For this review, take the finished solid that the model builds, in its own axes (mm). A direction names the side the tool comes from. Round coordinates to 2 decimals unless told otherwise and drop trailing zeros. Order: outer loops, then holes, each group sorted by start corner. A loop starts at its lowest first (then second) coordinate and runs counter-clockwise, first axis right, second up.
```python
from build123d import *

# Parameters (mm, degrees)
F0_R     = 3.302
F1_DEPTH = 6.35


with BuildPart() as f1:
    # F0 (on Top) → F1 (new body)
    with BuildSketch(Plane.XY):
        with BuildLine():
            ThreePointArc((12.499722, -2.252856), (12.650669, -1.13092), (12.701119, 0))
            ThreePointArc((12.701119, 0), (12.700826, 0.086204), (12.699949, 0.172405))
            ThreePointArc((12.699949, 0.172405), (12.657421, 1.052668), (12.553954, 1.927863))
            ThreePointArc((12.553954, 1.927863), (12.311527, 3.121654), (11.955851, 4.28673))
            ThreePointArc((11.955851, 4.28673), (11.629806, 5.105489), (11.24777, 5.899668))
            ThreePointArc((11.24777, 5.899668), (10.630855, 6.95006), (9.916151, 7.936522))
            ThreePointArc((9.916151, 7.936522), (9.341922, 8.605052), (8.722716, 9.232153))
            ThreePointArc((8.722716, 9.232153), (7.798165, 10.02532), (6.801882, 10.726268))
            ThreePointArc((6.801882, 10.726268), (6.041695, 11.172123), (5.25242, 11.564191))
            ThreePointArc((5.25242, 11.564191), (4.120423, 12.01418), (2.950524, 12.353656))
            ThreePointArc((2.950524, 12.353656), (2.086757, 12.528522), (1.212943, 12.643069))
            ThreePointArc((1.212943, 12.643069), (0.607166, 12.686598), (0, 12.701119))
            ThreePointArc((0, 12.701119), (-0.610992, 12.686414), (-1.22057, 12.642335))
            ThreePointArc((-1.22057, 12.642335), (-2.094314, 12.527261), (-2.957976, 12.351874))
            ThreePointArc((-2.957976, 12.351874), (-4.12767, 12.011693), (-5.259395, 11.56102))
            ThreePointArc((-5.259395, 11.56102), (-6.048433, 11.168477), (-6.808351, 10.722163))
            ThreePointArc((-6.808351, 10.722163), (-7.804211, 10.020614), (-8.728284, 9.226889))
            ThreePointArc((-8.728284, 9.226889), (-9.347111, 8.599415), (-9.920937, 7.930538))
            ThreePointArc((-9.920937, 7.930538), (-10.635046, 6.943646), (-11.251327, 5.892882))
            ThreePointArc((-11.251327, 5.892882), (-11.632884, 5.098473), (-11.958434, 4.279517))
            ThreePointArc((-11.958434, 4.279517), (-12.313408, 3.114226), (-12.555115, 1.920289))
            ThreePointArc((-12.555115, 1.920289), (-12.658054, 1.045032), (-12.70005, 0.164744))
            ThreePointArc((-12.70005, 0.164744), (-12.657421, -1.052668), (-12.498361, -2.260396))
            ThreePointArc((-12.498361, -2.260396), (-12.311527, -3.121654), (-12.065419, -3.967882))
            ThreePointArc((-12.065419, -3.967882), (-11.629806, -5.105489), (-11.087216, -6.196133))
            ThreePointArc((-11.087216, -6.196133), (-10.630855, -6.95006), (-10.123312, -7.670526))
            ThreePointArc((-10.123312, -7.670526), (-9.341922, -8.605052), (-8.474599, -9.460423))
            ThreePointArc((-8.474599, -9.460423), (-7.798165, -10.02532), (-7.084187, -10.54195))
            ThreePointArc((-7.084187, -10.54195), (-6.041695, -11.172123), (-4.943627, -11.699528))
            ThreePointArc((-4.943627, -11.699528), (-4.120423, -12.01418), (-3.27738, -12.27099))
            ThreePointArc((-3.27738, -12.27099), (-2.086757, -12.528522), (-0.876937, -12.670809))
            ThreePointArc((-0.876937, -12.670809), (0.003831, -12.701118), (0.884581, -12.670278))
            ThreePointArc((0.884581, -12.670278), (2.094314, -12.527261), (3.284782, -12.269011))
            ThreePointArc((3.284782, -12.269011), (4.12767, -12.011693), (4.950684, -11.696544))
            ThreePointArc((4.950684, -11.696544), (6.048433, -11.168477), (7.090545, -10.537675))
            ThreePointArc((7.090545, -10.537675), (7.804211, -10.020614), (8.480304, -9.455308))
            ThreePointArc((8.480304, -9.455308), (9.347111, -8.599415), (10.127937, -7.664418))
            ThreePointArc((10.127937, -7.664418), (10.635046, -6.943646), (11.090952, -6.189443))
            ThreePointArc((11.090952, -6.189443), (11.632884, -5.098473), (12.06781, -3.960603))
            ThreePointArc((12.06781, -3.960603), (12.313408, -3.114226), (12.499722, -2.252856))
        make_face()
        Circle(F0_R, mode=Mode.SUBTRACT)
        with BuildLine():
            ThreePointArc((12.699949, 0.172405), (12.700826, 0.086204), (12.701119, 0))
            ThreePointArc((12.701119, 0), (12.650669, -1.13092), (12.499722, -2.252856))
            Line((12.499722, -2.252856), (14.69304, -1.2175))
            Line((14.69304, -1.2175), (12.699949, 0.172405))
        make_face()
        with BuildLine():
            ThreePointArc((11.955851, 4.28673), (12.311527, 3.121654), (12.553954, 1.927863))
            Line((12.553954, 1.927863), (14.292252, 3.61929))
            Line((14.292252, 3.61929), (11.955851, 4.28673))
        make_face()
        with BuildLine():
            Line((13.501609, -5.922355), (12.06781, -3.960603))
            ThreePointArc((12.06781, -3.960603), (11.632884, -5.098473), (11.090952, -6.189443))
            Line((11.090952, -6.189443), (13.501609, -5.922355))
        make_face()
        with BuildLine():
            ThreePointArc((9.916151, 7.936522), (10.630855, 6.95006), (11.24777, 5.899668))
            Line((11.24777, 5.899668), (12.342677, 8.063873))
            Line((12.342677, 8.063873), (9.916151, 7.936522))
        make_face()
        with BuildLine():
            Line((10.847069, -9.98543), (10.127937, -7.664418))
            ThreePointArc((10.127937, -7.664418), (9.347111, -8.599415), (8.480304, -9.455308))
            Line((8.480304, -9.455308), (10.847069, -9.98543))
        make_face()
        with BuildLine():
            ThreePointArc((6.801882, 10.726268), (7.798165, 10.02532), (8.722716, 9.232153))
            Line((8.722716, 9.232153), (9.055581, 11.634611))
            Line((9.055581, 11.634611), (6.801882, 10.726268))
        make_face()
        with BuildLine():
            Line((7.017081, -12.96643), (7.090545, -10.537675))
            ThreePointArc((7.090545, -10.537675), (6.048433, -11.168477), (4.950684, -11.696544))
            Line((4.950684, -11.696544), (7.017081, -12.96643))
        make_face()
        with BuildLine():
            ThreePointArc((2.950524, 12.353656), (4.120423, 12.01418), (5.25242, 11.564191))
            Line((5.25242, 11.564191), (4.787173, 13.944558))
            Line((4.787173, 13.944558), (2.950524, 12.353656))
        make_face()
        with BuildLine():
            Line((2.426683, -14.542315), (3.284782, -12.269011))
            ThreePointArc((3.284782, -12.269011), (2.094314, -12.527261), (0.884581, -12.670278))
            Line((0.884581, -12.670278), (2.426683, -14.542315))
        make_face()
        with BuildLine():
            ThreePointArc((0, 12.701119), (0.607166, 12.686598), (1.212943, 12.643069))
            Line((1.212943, 12.643069), (0, 14.743396))
            Line((0, 14.743396), (0, 12.701119))
        make_face()
        with BuildLine():
            Line((-2.426683, -14.542315), (-0.876937, -12.670809))
            ThreePointArc((-0.876937, -12.670809), (-2.086757, -12.528522), (-3.27738, -12.27099))
            Line((-3.27738, -12.27099), (-2.426683, -14.542315))
        make_face()
        with BuildLine():
            ThreePointArc((-1.22057, 12.642335), (-0.610992, 12.686414), (0, 12.701119))
            Line((0, 12.701119), (0, 14.743396))
            Line((0, 14.743396), (-1.22057, 12.642335))
        make_face()
        with BuildLine():
            Line((-7.017081, -12.96643), (-4.943627, -11.699528))
            ThreePointArc((-4.943627, -11.699528), (-6.041695, -11.172123), (-7.084187, -10.54195))
            Line((-7.084187, -10.54195), (-7.017081, -12.96643))
        make_face()
        with BuildLine():
            ThreePointArc((-5.259395, 11.56102), (-4.12767, 12.011693), (-2.957976, 12.351874))
            Line((-2.957976, 12.351874), (-4.787173, 13.944558))
            Line((-4.787173, 13.944558), (-5.259395, 11.56102))
        make_face()
        with BuildLine():
            Line((-10.847069, -9.98543), (-8.474599, -9.460423))
            ThreePointArc((-8.474599, -9.460423), (-9.341922, -8.605052), (-10.123312, -7.670526))
            Line((-10.123312, -7.670526), (-10.847069, -9.98543))
        make_face()
        with BuildLine():
            ThreePointArc((-8.728284, 9.226889), (-7.804211, 10.020614), (-6.808351, 10.722163))
            Line((-6.808351, 10.722163), (-9.055581, 11.634611))
            Line((-9.055581, 11.634611), (-8.728284, 9.226889))
        make_face()
        with BuildLine():
            Line((-13.501609, -5.922355), (-11.087216, -6.196133))
            ThreePointArc((-11.087216, -6.196133), (-11.629806, -5.105489), (-12.065419, -3.967882))
            Line((-12.065419, -3.967882), (-13.501609, -5.922355))
        make_face()
        with BuildLine():
            ThreePointArc((-11.251327, 5.892882), (-10.635046, 6.943646), (-9.920937, 7.930538))
            Line((-9.920937, 7.930538), (-12.342677, 8.063873))
            Line((-12.342677, 8.063873), (-11.251327, 5.892882))
        make_face()
        with BuildLine():
            Line((-14.69304, -1.2175), (-12.498361, -2.260396))
            ThreePointArc((-12.498361, -2.260396), (-12.657421, -1.052668), (-12.70005, 0.164744))
            Line((-12.70005, 0.164744), (-14.69304, -1.2175))
        make_face()
        with BuildLine():
            ThreePointArc((-12.555115, 1.920289), (-12.313408, 3.114226), (-11.958434, 4.279517))
            Line((-11.958434, 4.279517), (-14.292252, 3.61929))
            Line((-14.292252, 3.61929), (-12.555115, 1.920289))
        make_face()
    extrude(amount=F1_DEPTH)


solid = f1.part
```
Q1. Mouldability with a two-part tool opening along Y and no side actions: class faces 5 (the face through (5.023, 12.738, 3.131)), 6 (the face through (8.887, 10.417, 3.131)), 7 (the face through (2.85, -13.42, 3.13)) as +Y half, -Y half, draft (parallel to the pull), parting line (faces both ways), or undercut.
Q2. Take a section at A-A, the plane y = -5.25. State the section outline as (x, z) points.
Q3. Clearance check with flat-ended pins moving along their axes: pin 1 (1.5 mm diameter, centred on y = 10, z = 1.5, fed in from +X); pin 2 (1 mm diameter, centred on x = -8.5, z = 4.5, fed in from +Y); pin 3 (1 mm diameter, centred on x = 2.5, z = 1.5, fed in from +Y). State where each tip first meets the part, or that it passes through.
Q4. Wall thickness on line 1 (Y direction, x = -13, z = 5); line 2 (Y direction, x = -1.5, z = 1.5); line 3 (Y direction, x = 6.75, z = 4.25): over which ranges is each line inside the solid? List them lowest first.
Q5. Take a section at B-B, the plane y = -11.25. State the section outline as (x, z) points.
Q6. Tool access review of faces 1 (the face through (11.635, 5.094, 3.131)), 2 (the face through (-12.77, -4.93, 3.13)), 3 (the face through (1.64, -13.59, 3.13)), 4 (the face through (-6.038, 11.174, 3.131)): name each direction out of +Z, -Z, +X, -X, +Y, -Y from which nothing blocks a thin tool from reaching the whole face with its end or side.
Working result:
1. face 5: +Y half
1. face 6: undercut
1. face 7: -Y half
2. outline: (-13.01, 0) - (13.01, 0) - (13.01, 6.35) - (-13.01, 6.35) - close
3. pin 1: stops at x = 8.93
3. pin 2: stops at y = 11.61
3. pin 3: stops at y = 12.54
4. line 1: y = -5.98 to -5.24, -2.02 to -0.04, 2.36 to 3.98
4. line 2: y = -13.42 to -2.94, 2.94 to 12.61
4. line 3: y = -12.8 to 10.76
5. outline: (-7.06, 0) - (7.07, 0) - (7.07, 6.35) - (-7.06, 6.35) - close
6. face 1: +Z, -Z, +X
6. face 2: +Z, -Z, -X
6. face 3: +Z, -Z, -Y
6. face 4: +Z, -Z, +Y
